Can you work these out from the model? Positions are in its coordinate system, mm. Face numbers are marked on the shaded views. A direction names the side the tool comes from. Round coordinates to 2 decimals unless told otherwise and drop trailing zeros. Loops run counter-clockwise (first coordinate to the right, second up) from the corner with the lowest first, then second, coordinate; pieces in that order, holes last. Notation, with made-up numbers: M 25.5,31.25 L 66.5,31.25 A14 cw 66.5,57.25 Z; hole C 73.25,74.5 d5. An arc over 180 degrees is marked long. Return JSON: item names as keys, results as strings.
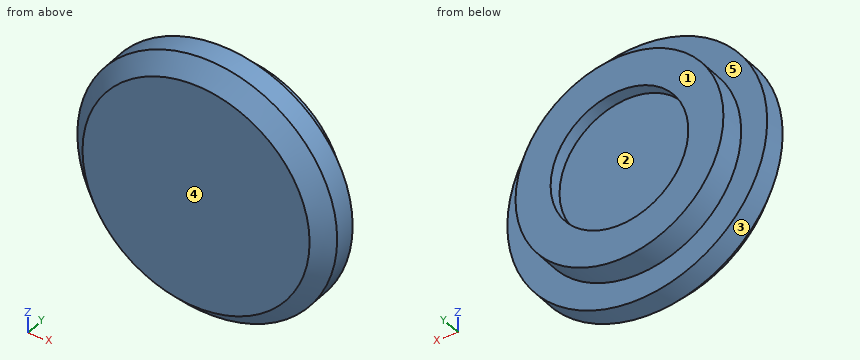
```python
from build123d import *

# Parameters (mm, degrees)
F0_R     = 12.7
F0_R_2   = 10.16
F0_R_3   = 6.731
F1_DEPTH = 6.35
F2_DEPTH = 2.54
F3_DEPTH = 1.27
F4_SIZE  = 1.6002


with BuildPart() as f1:
    # F0 (on Front) → F1 (new body)
    with BuildSketch(Plane.XZ):
        Circle(F0_R)
        Circle(F0_R_2, mode=Mode.SUBTRACT)
        Circle(F0_R_2)
        Circle(F0_R_3, mode=Mode.SUBTRACT)
        Circle(F0_R_3)
    extrude(amount=F1_DEPTH)

    # F0 (on Front) → F2 (cut)
    with BuildSketch(Plane.XZ):
        Circle(F0_R)
        Circle(F0_R_2, mode=Mode.SUBTRACT)
    extrude(amount=F2_DEPTH, mode=Mode.SUBTRACT)

    # F0 (on Front) → F3 (cut)
    with BuildSketch(Plane.XZ):
        Circle(F0_R_3)
    extrude(amount=F3_DEPTH, mode=Mode.SUBTRACT)

    # F4
    f4_edges = [f1.edges().sort_by_distance(p)[0] for p in [
        (-12.7, -6.35, 0),
    ]]
    chamfer(f4_edges, length=F4_SIZE)


solid = f1.part
```
Q1. If I drill on line 1 along Z through (x, y) = (0, -0.45); line 2 along Y through (x, z) = (-7, -7.5); line 3 along X through (y, z) = (-0.25, 3.5), over which ranges is the centre line in solid material (lowest first)?
Results:
{"line 1": "z = -10.16 to -6.73, 6.73 to 10.16", "line 2": "y = -6.35 to -2.54", "line 3": "x = -9.54 to -5.75, 5.75 to 9.54"}
Q2. Suppose I cut it at D-D, the plane y = -2. Please give me the cut outline in (x, z).
Results:
{"outline": "C 0,0 d20.32"}
Q3. On a 3-axis mill with a long thin cutter (end or side, diameter ignored), from which of +Z, -Z, +X, -X, +Y, -Y can I reach the whole of each face in a straight line? I mean the marked faces 4 and 5. Say none if no direction works.
Results:
{"face 4": "+Z, -Z, +X, -X, -Y", "face 5": "+Y"}
Q4. Thinking about a two-plate mould opening in X: for the marked faces 1, 2 and 3, which applies, pulls with the +X half, pulls with the -X half, needs draft (parallel to the pull), parting line crosses it, or undercut?
Results:
{"face 1": "needs draft", "face 2": "undercut", "face 3": "parting line crosses it"}
Q5. I'm going to push flat-ended pins straight in: pin 1 Ø6.5 at (x, z) = (-1.5, 1.5) entering from +Y; pin 2 Ø2 at (x, y) = (-9.5, -1.5) entering from -Z; pin 3 Ø2 at (y, z) = (-5, 4) entering from -X. Where does each tip first touch, or does it pass through?
Results:
{"pin 1": "stops at y = -1.27", "pin 2": "stops at z = -5.57", "pin 3": "stops at x = -12.33"}
Q6. Suppose I cut it at B-B, the plane y = -0.5. Please give me the cut outline in (x, z).
Results:
{"outline": "C 0,0 d20.32; hole C 0,0 d13.46"}
Q7. Suppose I cut it at C-C, the plane z = 0. Please give me the cut outline in (x, y).
Results:
{"outline": "M -12.7,-4.75 L -11.1,-6.35 L 11.1,-6.35 L 12.7,-4.75 L 12.7,-2.54 L 10.16,-2.54 L 10.16,0 L 6.73,0 L 6.73,-1.27 L -6.73,-1.27 L -6.73,0 L -10.16,0 L -10.16,-2.54 L -12.7,-2.54 Z"}
Q8. Suppose I cut it at A-A, the plane x = 0. Please give me the cut outline in (y, z), plus the area to 3 significant figures.
Results:
{"outline": "M -6.35,-11.1 L -4.75,-12.7 L -2.54,-12.7 L -2.54,-10.16 L 0,-10.16 L 0,-6.73 L -1.27,-6.73 L -1.27,6.73 L 0,6.73 L 0,10.16 L -2.54,10.16 L -2.54,12.7 L -4.75,12.7 L -6.35,11.1 Z", "area": "129 mm2"}
